Build history of the part. All positions in model axes, mm. A direction names the side the tool comes from. Give positions to 0.01 mm unless a question says otherwise; leave off trailing zeros. Write each loop counter-clockwise with the first axis right and the second up, starting at its lowest first coordinate (ties: lowest second). Pieces come first, ordered by that corner, then holes. Notation, with made-up numbers: M -21,21 L 17,21 A20 ccw 17,28 Z; hole C -29.5,78 d8. An arc over 180 degrees is marked long. One line per item, written item: value. Start each with the question number.
from build123d import *

# Parameters (mm, degrees)
SKETCH1_W             = 20
SKETCH1_H             = 7
BOSS_EXTRUDE1_DEPTH   = 6
SKETCH234_W           = 10
SKETCH234_H           = 6
BOSS_EXTRUDE234_DEPTH = 6
FILLET134_R           = 1
M3_CLEARANCE_HOLE1_D  = 3.2
FILLET135_R           = 5


with BuildPart() as part:
    # Sketch1 → Boss-Extrude1 (new body)
    with BuildSketch(Plane(origin=(0, 0, 0), x_dir=(1, 0, 0), z_dir=(0, 1, 0))):
        Rectangle(SKETCH1_W, SKETCH1_H)
    extrude(amount=BOSS_EXTRUDE1_DEPTH)

    # Sketch234 → Boss-Extrude234 (add)
    with BuildSketch(Plane(origin=(0.767778608, 0, -3.5), x_dir=(-1, 0, 0), z_dir=(0, 0, -1))):
        with Locations((0.767778608, 3)):
            Rectangle(SKETCH234_W, SKETCH234_H)
    extrude(amount=BOSS_EXTRUDE234_DEPTH)

    # Fillet134
    fillet134_edges = [part.edges().sort_by_distance(p)[0] for p in [
        (5, 3, -9.5),
        (-5, 3, -9.5),
    ]]
    fillet(fillet134_edges, radius=FILLET134_R)

    # M3 Clearance Hole1 (through all)
    with Locations(Plane(origin=(0, 6, 0), x_dir=(1, 0, 0), z_dir=(0, 1, 0))):
        with Locations((-5, 0), (5, 0)):
            Hole(M3_CLEARANCE_HOLE1_D / 2)

    # Fillet135
    fillet135_edges = [part.edges().sort_by_distance(p)[0] for p in [
        (10, 3, 3.5),
        (-10, 3, 3.5),
    ]]
    fillet(fillet135_edges, radius=FILLET135_R)


solid = part.part
1) Mould opens along X. For faces 4 (the face through (10, 3, -2)), 5 (the face through (6.6, 2.96, -0.07)), 6 (the face through (-4.715, 3.042, -9.199)) say: released by +X, released by -X, zero draft, split by the parting line, or undercut.
2) Band-saw the part on A-A (y = 2.85). List the corners of the cut face in (x, z).
3) Band-saw the part on B-B (z = 0). List the corners of the cut face in (x, y).
4) Tool access for faces 1 (the face through (5, 3, -6)), 2 (the face through (-5, 3, -6)), 3 (the face through (0, 3, 3.5)): list every direction of +Z, -Z, +X, -X, +Y, -Y with a clear straight run to the whole face (end or side of a thin tool).
5) Band-saw the part on C-C (x = -3.75). List the corners of the cut face in (y, z), then the cut area to 3 significant figures.
6) Probe line 1 along X through (y, z) = (1.15, -8); line 2 along X through (y, z) = (2.35, -0.5); line 3 along X through (y, z) = (0.4, 0.5). List the from-to ranges inside material, lowest first. Write a range as from..to.
7) Drop flat-ended pins along their axis: P1, Ø3, axis at y = 3, z = 0.5, coming from the -X side; P2, Ø1.9, axis at x = 5, z = 0, coming from the -Y side; P3, Ø2.5, axis at y = 2, z = -5.5, coming from the +X side. Give the stop position or say it passes through.
8) Band-saw the part on D-D (z = -5.25). List the corners of the cut face in (x, y), then the cut area to 3 significant figures.
Model answer:
1. face 4: released by +X
1. face 5: undercut
1. face 6: released by -X
2. outline: M -10,-3.5 L -5,-3.5 L -5,-8.5 A1 ccw -4,-9.5 L 4,-9.5 A1 ccw 5,-8.5 L 5,-3.5 L 10,-3.5 L 10,-1.5 A5 ccw 5,3.5 L -5,3.5 A5 ccw -10,-1.5 Z; hole C -5,0 d3.2; hole C 5,0 d3.2
3. outline: M -9.77,0 L -6.6,0 L -6.6,6 L -9.77,6 Z; M -3.4,0 L 3.4,0 L 3.4,6 L -3.4,6 Z; M 6.6,0 L 9.77,0 L 9.77,6 L 6.6,6 Z
4. face 1: -Z, +X, +Y, -Y
4. face 2: -Z, -X, +Y, -Y
4. face 3: +Z, +X, -X, +Y, -Y
5. outline: M 0,-9.5 L 6,-9.5 L 6,-1 L 0,-1 Z; M 0,1 L 6,1 L 6,3.5 L 0,3.5 Z
5. area: 66.0 mm²
6. line 1: x = -5..5
6. line 2: x = -9.9..-6.52, -3.48..3.48, 6.52..9.9
6. line 3: x = -9.58..-6.52, -3.48..3.48, 6.52..9.58
7. P1: stops at x = -9.97
7. P2: passes through
7. P3: stops at x = 5
8. outline: M -5,0 L 5,0 L 5,6 L -5,6 Z
8. area: 60.0 mm²
